The figure shows three views and two pictorial views of one solid part (mm, origin at its lowest corner). Answer the questions. A direction names the side the tool comes from. Round coordinates to 2 decimals unless told otherwise and drop trailing zeros. Order: outer loops, then holes, each group sorted by start corner. A loop starts at its lowest first (then second) coordinate and runs counter-clockwise, first axis right, second up. Notation, with made-up numbers: (66.25, 85.5) -> (105.25, 85.5) arc R29 ccw to (105.25, 116.5) -> close; hole circle Ø10 at (-39.75, -26). An arc over 180 degrees is marked (long way). Return JSON: item names as keys, results as strings. Group by question number.
(1) The part is cut by section B-B (z = 10). Determine the outline of the cut face in (x, y), plus the area to 3 significant figures.
(2) The part is cut by section C-C (y = 28). Determine the outline of the cut face in (x, z), plus the area to 3 significant figures.
(3) Each of these flat-tipped pins is pushed along its axis until it touches: pin 1 (1.5 mm diameter, centred on x = 5, y = 52, fed in from +Z); pin 2 (8 mm diameter, centred on x = 4.5, y = 26.5, fed in from +Z); pin 3 (4 mm diameter, centred on x = 2, z = 11, fed in from +Y). Where does it stop, or does it pass through?
(4) Consider line 1 (Y direction, x = 15.5, z = 12.5); line 2 (Y direction, x = 7.75, z = 18); line 3 (X direction, y = 37.5, z = 4). Determine where each line is inside the solid, lowest interval first. Write a range as [from, to].
(5) The part is cut by section D-D (z = 3.5). Determine the outline of the cut face in (x, y), plus the area to 3 significant figures.
(6) The part is cut by section A-A (x = 10). Determine the outline of the cut face in (y, z), plus the area to 3 significant figures.
(7) Which of the six approach directions +Z, -Z, +X, -X, +Y, -Y give full straight-line access (tool end or side, diameter ignored) to the marked faces 1 and 2?
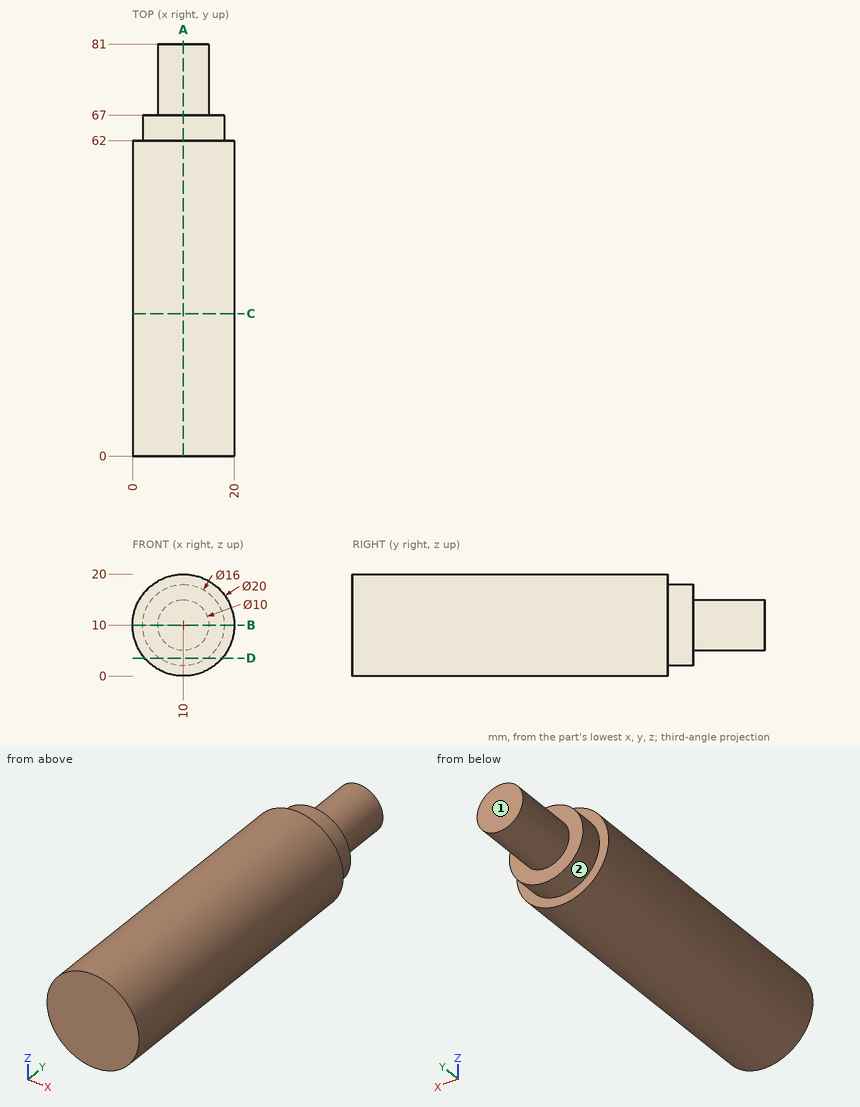
Answer below:
{
 "1": {"outline": "(0, 0) -> (20, 0) -> (20, 62) -> (18, 62) -> (18, 67) -> (15, 67) -> (15, 81) -> (5, 81) -> (5, 67) -> (2, 67) -> (2, 62) -> (0, 62) -> close", "area": "1,460 mm²"},
 "2": {"outline": "circle Ø20 at (10, 10)", "area": "314 mm²"},
 "3": {"pin 1": "stops at z = 19.05", "pin 2": "stops at z = 19.89", "pin 3": "stops at y = 67"},
 "4": {"line 1": "y = [0, 67]", "line 2": "y = [0, 62]", "line 3": "x = [2, 18]"},
 "5": {"outline": "(2.4, 0) -> (17.6, 0) -> (17.6, 62) -> (14.66, 62) -> (14.66, 67) -> (5.34, 67) -> (5.34, 62) -> (2.4, 62) -> close", "area": "989 mm²"},
 "6": {"outline": "(0, 0) -> (62, 0) -> (62, 2) -> (67, 2) -> (67, 5) -> (81, 5) -> (81, 15) -> (67, 15) -> (67, 18) -> (62, 18) -> (62, 20) -> (0, 20) -> close", "area": "1,460 mm²"},
 "7": {"face 1": "+Z, -Z, +X, -X, +Y", "face 2": "+Y"}
}
